Answer from the drawing. Dimensions are ordinates in mm from the lowest x, y and z of the part. A direction names the side the tool comes from. Give positions to 0.01 mm unless a question says otherwise; leave off trailing zeros. Loops run counter-clockwise (first coordinate to the right, second up) from the corner with the lowest first, then second, coordinate; pieces in that order, holes last. Notation, with made-up numbers: M 69.5,-29 L 109.5,-29 A27 cw 109.5,-3 Z; hole C 47.25,83 d5. An arc over 180 degrees is marked long. Use a Markdown table: item, result.
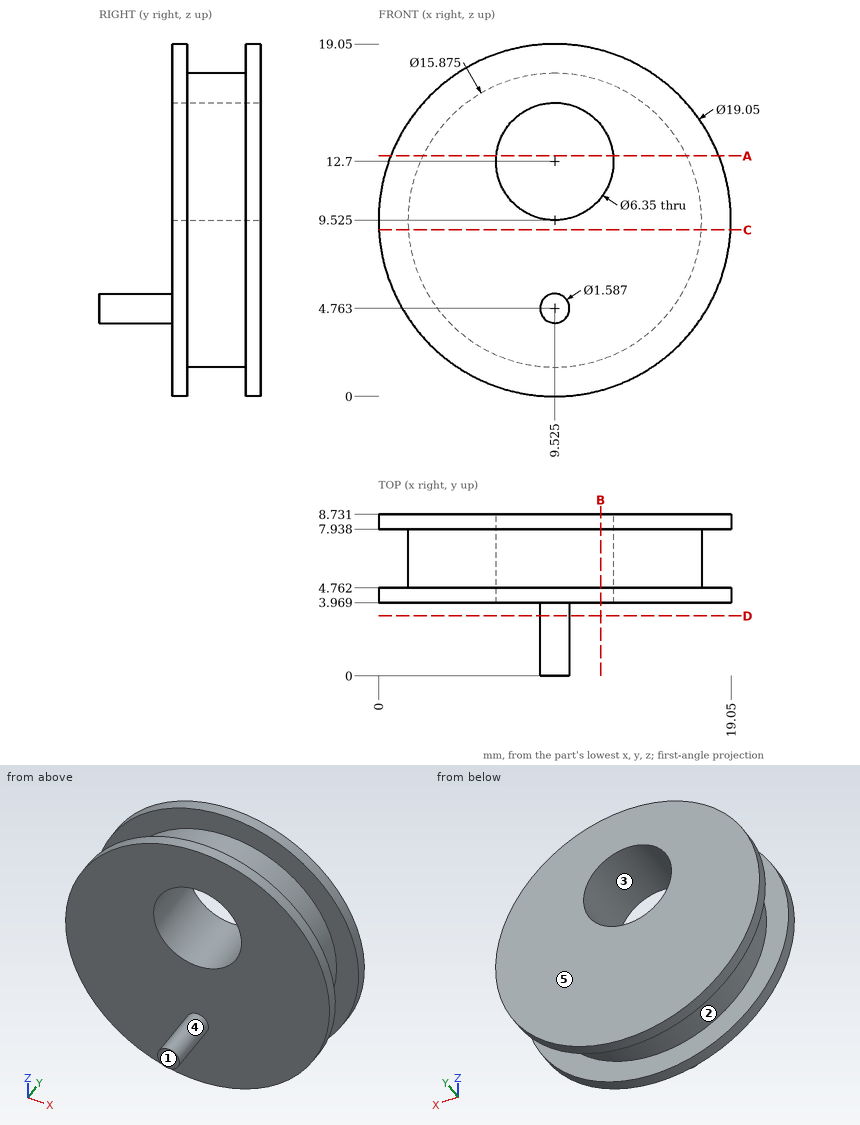
(1) A cutting plane is placed at C-C (z = 9). Write down the section's boundary in (x, y) (1 decimal).
Entries:
| item | result |
|---|---|
| outline | M 0,4 L 19,4 L 19,4.8 L 17.4,4.8 L 17.4,7.9 L 19,7.9 L 19,8.7 L 0,8.7 L 0,7.9 L 1.6,7.9 L 1.6,4.8 L 0,4.8 Z |
(2) Given P1, Ø1, axis at y = 5, z = 14, coming from the -X side; P2, Ø1.5, axis at x = 9.5, z = 6.5, coming from the -Y side; P3, Ø1.5, axis at x = 5.5, y = 7, coming from the +Z side (1 decimal), each flat-ended and moving along its own axis, determine where each tip first touches the part or whether it passes through.
Entries:
| item | result |
|---|---|
| P1 | stops at x = 0.9 |
| P2 | stops at y = 3.97 |
| P3 | stops at z = 16.8 |
(3) A cutting plane is placed at B-B (x = 12). Write down the section's boundary in (y, z).
Entries:
| item | result |
|---|---|
| outline | M 3.97,0.33 L 4.76,0.33 L 4.76,1.98 L 7.94,1.98 L 7.94,0.33 L 8.73,0.33 L 8.73,10.71 L 3.97,10.71 Z; M 3.97,14.69 L 8.73,14.69 L 8.73,18.72 L 7.94,18.72 L 7.94,17.07 L 4.76,17.07 L 4.76,18.72 L 3.97,18.72 Z |
(4) Consider probe 1 along Y at (x, z) = (2, 6); probe 2 along Z at (x, y) = (9.5, 7.5) (1 decimal); probe 3 along Y at (x, z) = (7.25, 2.25). Determine where each line is inside the solid, lowest interval first. Write a range as [from, to].
Entries:
| item | result |
|---|---|
| probe 1 | y = [3.97, 4.76], [7.94, 8.73] |
| probe 2 | z = [1.6, 9.5], [15.9, 17.5] |
| probe 3 | y = [3.97, 8.73] |
(5) A cutting plane is placed at A-A (z = 13). Write down the section's boundary in (x, y) (1 decimal).
Entries:
| item | result |
|---|---|
| outline | M 0.7,4 L 6.4,4 L 6.4,8.7 L 0.7,8.7 L 0.7,7.9 L 2.4,7.9 L 2.4,4.8 L 0.7,4.8 Z; M 12.7,4 L 18.4,4 L 18.4,4.8 L 16.7,4.8 L 16.7,7.9 L 18.4,7.9 L 18.4,8.7 L 12.7,8.7 Z |
(6) Which of the six approach directions +Z, -Z, +X, -X, +Y, -Y give full straight-line access (tool end or side, diameter ignored) to the marked faces 1 and 2?
Entries:
| item | result |
|---|---|
| face 1 | +Z, -Z, +X, -X, -Y |
| face 2 | none |
(7) A cutting plane is placed at D-D (y = 3.25). Write down the section's boundary in (x, z) (1 decimal).
Entries:
| item | result |
|---|---|
| outline | C 9.5,4.8 d1.6 |
(8) The mould has two halves that part along X. Classify the marked faces 3, 4 and 5: released by +X, released by -X, zero draft, split by the parting line, or undercut.
Entries:
| item | result |
|---|---|
| face 3 | undercut |
| face 4 | split by the parting line |
| face 5 | zero draft |
